from build123d import *

# Parameters (mm, degrees)
F1_DEPTH = 60
F3_DEPTH = 60
F4_R     = 2


with BuildPart() as f1:
    # F0 (on Front) → F1 (new body)
    with BuildSketch(Plane.XZ):
        Polygon((-125, 0), (0, 0), (125, 0), (125, 150), (-125, 150), align=None)
    extrude(amount=F1_DEPTH)

    # F2 (on Front) → F3 (cut)
    with BuildSketch(Plane.XZ):
        Polygon((-67.3774927855, 46.4679524302), (-75.1930549741, 0), (75.1930549741, 0), (67.3774927855, 46.4679524302), (31.8278856575, 55.0686642528), (0, 74.5636075735), (-31.8278856575, 55.0686642528), align=None)
    extrude(amount=F3_DEPTH, mode=Mode.SUBTRACT)

    # F4
    f4_edges = [f1.edges().sort_by_distance(p)[0] for p in [
        (-125, -60, 75),
        (0, -60, 150),
        (125, -60, 75),
        (-125, -30, 150),
        (125, -30, 150),
        (0, 0, 150),
        (-125, 0, 75),
        (-125, -30, 0),
        (125, 0, 75),
        (125, -30, 0),
        (100.096527, 0, 0),
        (75.193055, -30, 0),
        (100.096527, -60, 0),
        (-100.096527, -60, 0),
        (-71.285274, -60, 23.233976),
        (-49.602689, -60, 50.768308),
        (-15.913943, -60, 64.816136),
        (31.827886, -30, 55.068664),
        (-31.827886, -30, 55.068664),
        (0, -30, 74.563608),
        (15.913943, -60, 64.816136),
        (49.602689, -60, 50.768308),
        (67.377493, -30, 46.467952),
        (71.285274, -60, 23.233976),
        (-100.096527, 0, 0),
        (-75.193055, -30, 0),
        (71.285274, 0, 23.233976),
        (15.913943, 0, 64.816136),
        (49.602689, 0, 50.768308),
        (-15.913943, 0, 64.816136),
        (-49.602689, 0, 50.768308),
        (-71.285274, 0, 23.233976),
    ]]
    fillet(f4_edges, radius=F4_R)


solid = f1.part
Work out the finished part from the listing and answer in its coordinate system (mm). A direction names the side the tool comes from. Coordinates: 2 decimals unless noted, no trailing zeros. Loops run counter-clockwise (first coordinate to the right, second up) from the corner with the lowest first, then second, coordinate; pieces in that order, holes last. Notation, with made-up numbers: (52.25, -38.5) -> (76.25, -38.5) arc R26 ccw to (76.25, -15.5) -> close; hole circle Ø3 at (8.5, -5.75). An arc over 180 degrees is marked (long way). Write each question's results on one line, items separated by ' | '. Start each with the question number.
1) Find section A-A on y = -18.5. Determine the outline of the cut face in (x, z).
2) For faces 4 (the flat face through (100, -30, 0)), 5 (the cylindrical face through (-71.68, -0.57, 24.5)), 6 (the flat face through (-2, 0, 92)), 7 (the cylindrical face through (49, -59.4, 51.5)), 8 (the flat face through (-49.51, -29.61, 50.79)), determine the directions among +Z, -Z, +X, -X, +Y, -Y from which every point of the face is accessible in a straight line to the end or side of a thin tool.
3) The mould has two halves that part along X. Classify faces 1 (the cylindrical face through (49, -0.6, 51.5)), 2 (the flat face through (-125, -30, 76)), 3 (the flat face through (-100, -30, 0)): pulls with the +X half, pulls with the -X half, needs draft (parallel to the pull), parting line crosses it, or undercut.
4) Consider line 1 along X through (y, z) = (-39, 32); line 2 along X through (y, z) = (-32, 38.5); line 3 along Z through (x, y) = (-24, -18). Determine where each line is inside the solid, lowest interval first.
5) Flat-ended cylindrical pins translate along their axes: P1, Ø1.5, axis at x = 32, y = -19.5, coming from the -Z side; P2, Ø10, axis at x = 3.5, y = -44.5, coming from the -Z side. Find the tip coordinate at first contact, or state that the pin passes through.
Response values:
1) outline: (-125, 2) arc R2 ccw to (-123, 0) -> (-76.88, 0) arc R2 ccw to (-74.91, 1.67) -> (-67.38, 46.47) -> (-32.13, 54.99) arc R2 ccw to (-31.56, 55.23) -> (-1.04, 73.92) arc R2 cw to (1.04, 73.92) -> (31.56, 55.23) arc R2 ccw to (32.13, 54.99) -> (66.09, 46.78) arc R2 cw to (67.6, 45.17) -> (74.91, 1.67) arc R2 ccw to (76.88, 0) -> (123, 0) arc R2 ccw to (125, 2) -> (125, 148) arc R2 ccw to (123, 150) -> (-123, 150) arc R2 ccw to (-125, 148) -> close
2) face 4: -Z, +X, -X, +Y, -Y | face 5: -Z, +Y | face 6: +Z, -Z, +X, -X, +Y | face 7: -Z, -Y | face 8: -Z, +Y, -Y
3) face 1: undercut | face 2: pulls with the -X half | face 3: needs draft
4) line 1: x = -125 to -69.81, 69.81 to 125 | line 2: x = -125 to -68.72, 68.72 to 125 | line 3: z = 59.86 to 150
5) P1: stops at z = 54.85 | P2: stops at z = 69.36
